from build123d import *

# Parameters (mm, degrees)
BOSS_EXTRUDE1_DEPTH      = 40
BOSS_EXTRUDE1_DEPTH_BACK = 40
SKETCH1_R                = 10
CUT_EXTRUDE1_START       = -20
CUT_EXTRUDE1_DEPTH       = 20
CUT_EXTRUDE2_START       = -20
CUT_EXTRUDE2_DEPTH       = 20
SKETCH6_R                = 30
BOSS_EXTRUDE2_DEPTH      = 10
FILLET2_R                = 5
SHELL1_START             = -15
SHELL1_OUTLINE_R         = 15
SHELL1_DEPTH             = 30
SHELL1_START_2           = -35
SHELL1_2_OUTLINE_W       = 60.710678118
SHELL1_2_OUTLINE_H       = 40
SHELL1_2_DEPTH           = 70
SHELL1_START_3           = 715
SHELL1_3_OUTLINE_R       = 25
SHELL1_3_DEPTH           = 10
SHELL1_START_4           = -30.355339059
SHELL1_4_DEPTH           = 60.710678118


with BuildPart() as part:
    # Sketch1 → Boss-Extrude1 (new, two sides: drawn at the far end of the back side and taken through both)
    with BuildSketch(Plane.XY.offset(-BOSS_EXTRUDE1_DEPTH_BACK)):
        with BuildLine():
            Line((-35.355339059, 570), (-35.355339059, 720))
            Line((-35.355339059, 720), (35.355339059, 720))
            Line((35.355339059, 720), (35.355339059, 570))
            ThreePointArc((35.355339059, 570), (0, 534.644660941), (-35.355339059, 570))
        make_face()
        with Locations(Location((0, 570, 0), (0, 0, 180))):
            Circle(SKETCH1_R, mode=Mode.SUBTRACT)
    extrude(amount=BOSS_EXTRUDE1_DEPTH + BOSS_EXTRUDE1_DEPTH_BACK)

    # Sketch2 → Cut-Extrude1 (cut)
    with BuildSketch(Plane.XY.offset(40).offset(CUT_EXTRUDE1_START)):
        with BuildLine():
            Line((-35.355339059, 570), (-35.355339059, 670))
            Line((-35.355339059, 670), (35.355339059, 670))
            Line((35.355339059, 670), (35.355339059, 570))
            ThreePointArc((35.355339059, 570), (0, 534.644660941), (-35.355339059, 570))
        make_face()
    extrude(amount=CUT_EXTRUDE1_DEPTH, mode=Mode.SUBTRACT)

    # Sketch3 → Cut-Extrude2 (cut)
    with BuildSketch(Plane(origin=(0, 0, -40), x_dir=(-1, 0, 0), z_dir=(0, 0, -1)).offset(CUT_EXTRUDE2_START)):
        with BuildLine():
            Line((-35.355339059, 570), (-35.355339059, 670))
            Line((-35.355339059, 670), (35.355339059, 670))
            Line((35.355339059, 670), (35.355339059, 570))
            ThreePointArc((35.355339059, 570), (0, 534.644660941), (-35.355339059, 570))
        make_face()
    extrude(amount=CUT_EXTRUDE2_DEPTH, mode=Mode.SUBTRACT)

    # Sketch6 → Boss-Extrude2 (add)
    with BuildSketch(Plane(origin=(0, 720, 0), x_dir=(1, 0, 0), z_dir=(0, 1, 0))):
        with Locations(Location((0, 0, 0), (0, 0, 270))):
            Circle(SKETCH6_R)
    extrude(amount=BOSS_EXTRUDE2_DEPTH)

    # Fillet2
    fillet2_edges = [part.edges().sort_by_distance(p)[0] for p in [
        (0, 720, -40),
        (0, 720, 40),
        (0, 670, 40),
        (0, 670, 20),
        (0, 670, -40),
        (0, 670, -20),
    ]]
    fillet(fillet2_edges, radius=FILLET2_R)

    # Shell1: read off the stored shape, not the designer's step
    # Shell1 outline → Shell1 (cut)
    with BuildSketch(Plane.XY.offset(SHELL1_START)):
        with BuildLine():
            ThreePointArc((-30.355339059, 570), (0, 539.644660941), (30.355339059, 570))
            Line((30.355339059, 570), (30.355339059, 715))
            Line((30.355339059, 715), (-30.355339059, 715))
            Line((-30.355339059, 715), (-30.355339059, 570))
        make_face()
        with Locations((0, 570)):
            Circle(SHELL1_OUTLINE_R, mode=Mode.SUBTRACT)
    extrude(amount=SHELL1_DEPTH, mode=Mode.SUBTRACT)

    # Shell1 2 outline → Shell1 2 (cut)
    with BuildSketch(Plane.XY.offset(SHELL1_START_2)):
        with Locations((0, 695)):
            Rectangle(SHELL1_2_OUTLINE_W, SHELL1_2_OUTLINE_H)
    extrude(amount=SHELL1_2_DEPTH, mode=Mode.SUBTRACT)

    # Shell1 3 outline → Shell1 3 (cut)
    with BuildSketch(Plane(origin=(0, 0, 0), x_dir=(1, 0, 0), z_dir=(0, 1, 0)).offset(SHELL1_START_3)):
        Circle(SHELL1_3_OUTLINE_R)
    extrude(amount=SHELL1_3_DEPTH, mode=Mode.SUBTRACT)

    # Shell1 4 outline → Shell1 4 (cut)
    with BuildSketch(Plane.YZ.offset(SHELL1_START_4)):
        with BuildLine():
            ThreePointArc((675, 25), (672.071067812, 17.928932188), (665, 15))
            Line((665, 15), (675, 15))
            Line((675, 15), (675, 25))
        make_face()
        with BuildLine():
            Line((675, -15), (665, -15))
            ThreePointArc((665, -15), (672.071067812, -17.928932188), (675, -25))
            Line((675, -25), (675, -15))
        make_face()
    extrude(amount=SHELL1_4_DEPTH, mode=Mode.SUBTRACT)


solid = part.part
Source: CAD feature listing. Evaluate the final solid. Frame: model axes, mm. A direction names the side the tool comes from. Give positions to 0.01 mm unless a question says otherwise; leave off trailing zeros. Order: outer loops, then holes, each group sorted by start corner. A loop starts at its lowest first (then second) coordinate and runs counter-clockwise, first axis right, second up. Notation, with made-up numbers: (86, 31.25) -> (106, 31.25) arc R12 cw to (106, 45.25) -> close; hole circle Ø5 at (29, 15). An arc over 180 degrees is marked (long way). Write item = value, one per line.
Item 1: Mould query, pull axis Z, two halves, no side actions, for faces 1 (the face through (0, 603, 15)), 2 (the face through (1.302, 560.085, -0.28)), 3 (the face through (0, 695, -40)). Classes: +Z half, -Z half, draft (parallel to the pull), parting line (faces both ways), or undercut.
Check result:
face_1 = undercut
face_2 = draft
face_3 = -Z half
Item 2: Section query C-C (x = -27). Output: boundary loops of the cut face in (y, z).
Check result:
outline = (547.17, -20) -> (665, -20) arc R5 cw to (670, -25) -> (670, -35) arc R5 ccw to (675, -40) -> (715, -40) arc R5 ccw to (720, -35) -> (720, -13.08) -> (730, -13.08) -> (730, 13.08) -> (720, 13.08) -> (720, 35) arc R5 ccw to (715, 40) -> (675, 40) arc R5 ccw to (670, 35) -> (670, 25) arc R5 cw to (665, 20) -> (547.17, 20) -> close; hole (556.13, -15) -> (665, -15) arc R10 cw to (675, -25) -> (675, -35) -> (715, -35) -> (715, 35) -> (675, 35) -> (675, 25) arc R10 cw to (665, 15) -> (556.13, 15) -> close
Item 3: Section query B-B (y = 660). Output: boundary loops of the cut face in (x, z).
Check result:
outline = (-35.36, -20) -> (35.36, -20) -> (35.36, 20) -> (-35.36, 20) -> close; hole (-30.36, -15) -> (30.36, -15) -> (30.36, 15) -> (-30.36, 15) -> close
Item 4: Section query D-D (x = -6). State how many separate pieces and enclosed holes the cut face has, then the cut area to 3 significant figures.
Check result:
separate_pieces = 2
enclosed_holes = 2
area = 2,780 mm²
Item 5: Ray query, probe 1 along X at (y, z) = (570, 1); probe 2 along Z at (x, y) = (-22, 595.5); probe 3 along X at (y, z) = (719, 0). Return the intervals inside material, ascending.
Check result:
probe_1 = -35.36 to -30.36, -15 to -10, 10 to 15, 30.36 to 35.36
probe_2 = -20 to -15, 15 to 20
probe_3 = -35.36 to -25, 25 to 35.36
Item 6: Contact query for flat-ended pins moving along their axis: pin 1 (21 mm diameter, centred on x = -1.5, y = 608, fed in from -Z); pin 2 (4 mm diameter, centred on x = 3.5, z = 25.5, fed in from -Y); pin 3 (3 mm diameter, centred on x = -21.5, y = 640, fed in from +Z); pin 4 (10 mm diameter, centred on y = 567, z = -6, fed in from +X). Output: stop coordinate, or through.
Check result:
pin_1 = -20
pin_2 = 669.77
pin_3 = 20
pin_4 = 35.36
Item 7: Set-up query: faces 4 (the face through (0, 725, 0)), 5 (the face through (0, 695, 40)), 6 (the face through (0, 720, 31)). Return all of +Z, -Z, +X, -X, +Y, -Y with unobstructed straight access to the full face (end or side cutting, diameter ignored); none if empty.
Check result:
face_4 = none
face_5 = +Z, +X, -X, +Y, -Y
face_6 = +Y
Item 8: Section query A-A (z = 0). Output: boundary loops of the cut face in (x, y), then the cut area to 3 significant figures.
Check result:
outline = (-35.36, 570) arc R35.36 ccw to (35.36, 570) -> (35.36, 720) -> (30, 720) -> (30, 730) -> (-30, 730) -> (-30, 720) -> (-35.36, 720) -> close; circle Ø30 at (0, 570); hole (-30.36, 570) arc R30.36 ccw to (30.36, 570) -> (30.36, 715) -> (25, 715) -> (25, 725) -> (-25, 725) -> (-25, 715) -> (-30.36, 715) -> close; hole circle Ø20 at (0, 570)
area = 2,810 mm²
